Part model, mm, in its own coordinate system. Face numbers are marked on the shaded views. A direction names the side the tool comes from. Coordinates: 2 decimals unless noted, no trailing zeros. Order: outer loops, then holes, each group sorted by start corner. A loop starts at its lowest first (then second) coordinate and runs counter-clockwise, first axis right, second up. Notation, with made-up numbers: (13.25, 61) - (48.25, 61) arc R29 ccw to (48.25, 92) - close; hole circle Ø10 at (-25, 80.25). An arc over 180 degrees is marked (long way). Use a Markdown table: item, result. Add a question column.
1) Saw through at C-C on z = -38.1. List the corners of the cut face in (x, y).
2) Saw through at A-A on y = 13.97. List the corners of the cut face in (x, z) (3 decimals), then the cut area to 3 significant figures.
3) Tool access for the marked faces 4 and 5: list every direction of +Z, -Z, +X, -X, +Y, -Y with a clear straight run to the whole face (end or side of a thin tool).
4) Two-plate mould, pull along Y, no slides. Class the marked faces 1, 2 and 3: +Y half, -Y half, draft (parallel to the pull), parting line (faces both ways), or undercut.
5) Drop a flat-ended pin along its axis: P1, Ø3.5, axis at x = 84.5, y = 15.5, coming from the +Z side. Give the stop position or say it passes through.
6) Saw through at B-B on x = 49. List the corners of the cut face in (y, z) (3 decimals).
7) Wall check: L1, parallel to Y at x = 89, z = -38.1; L2, parallel to Y at x = 69, z = -11 (3 decimals); L3, parallel to Z at x = 87, y = 16.25. Give the ranges that are in metal, low to high. Write a range as [from, to].
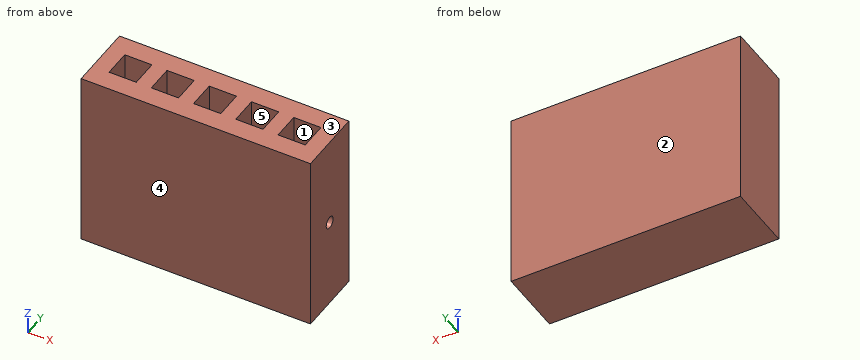
```python
from build123d import *

# Parameters (mm, degrees)
SKETCH1_W           = 96.52
SKETCH1_H           = 76.2
BOSS_EXTRUDE1_DEPTH = 27.94
SKETCH2_W           = 11.43
SKETCH2_H           = 11.43
CUT_EXTRUDE1_DEPTH  = 11.43
SKETCH3_R           = 2.5
CUT_EXTRUDE2_DEPTH  = 12.7


with BuildPart() as part:
    # Sketch1 → Boss-Extrude1 (new body)
    with BuildSketch(Plane(origin=(0, 0, 0), x_dir=(1, 0, 0), z_dir=(0, 1, 0))):
        with Locations((48.26, 38.1)):
            Rectangle(SKETCH1_W, SKETCH1_H)
    extrude(amount=BOSS_EXTRUDE1_DEPTH)

    # Sketch2 → Cut-Extrude1 (cut)
    with BuildSketch(Plane.XY):
        with Locations((12.7, 13.97)):
            Rectangle(SKETCH2_W, SKETCH2_H)
        with Locations((30.48, 13.97)):
            Rectangle(SKETCH2_W, SKETCH2_H)
        with Locations((48.26, 13.97)):
            Rectangle(SKETCH2_W, SKETCH2_H)
        with Locations((66.04, 13.97)):
            Rectangle(SKETCH2_W, SKETCH2_H)
        with Locations((83.82, 13.97)):
            Rectangle(SKETCH2_W, SKETCH2_H)
    extrude(amount=-CUT_EXTRUDE1_DEPTH, mode=Mode.SUBTRACT)

    # Sketch3 → Cut-Extrude2 (cut)
    with BuildSketch(Plane(origin=(96.52, 0, 0), x_dir=(0, 0, -1), z_dir=(1, 0, 0))):
        with Locations((38.1, 13.97)):
            Circle(SKETCH3_R)
    extrude(amount=-CUT_EXTRUDE2_DEPTH, mode=Mode.SUBTRACT)


solid = part.part
```
Results are:
| question | item | result |
|---|---|---|
| 1 | outline | (0, 0) - (96.52, 0) - (96.52, 11.47) - (83.82, 11.47) - (83.82, 16.47) - (96.52, 16.47) - (96.52, 27.94) - (0, 27.94) - close |
| 2 | outline | (0, -76.2) - (96.52, -76.2) - (96.52, -40.6) - (83.82, -40.6) - (83.82, -35.6) - (96.52, -35.6) - (96.52, 0) - (89.535, 0) - (89.535, -11.43) - (78.105, -11.43) - (78.105, 0) - (71.755, 0) - (71.755, -11.43) - (60.325, -11.43) - (60.325, 0) - (53.975, 0) - (53.975, -11.43) - (42.545, -11.43) - (42.545, 0) - (36.195, 0) - (36.195, -11.43) - (24.765, -11.43) - (24.765, 0) - (18.415, 0) - (18.415, -11.43) - (6.985, -11.43) - (6.985, 0) - (0, 0) - close |
| 2 | area | 6,640 mm2 |
| 3 | face 4 | +Z, -Z, +X, -X, -Y |
| 3 | face 5 | +Z |
| 4 | face 1 | undercut |
| 4 | face 2 | +Y half |
| 4 | face 3 | draft |
| 5 | P1 | z = -11.43 |
| 6 | outline | (0, -76.2) - (27.94, -76.2) - (27.94, 0) - (19.685, 0) - (19.685, -11.43) - (8.255, -11.43) - (8.255, 0) - (0, 0) - close |
| 7 | L1 | [0, 11.47], [16.47, 27.94] |
| 7 | L2 | [0, 8.255], [19.685, 27.94] |
| 7 | L3 | [-76.2, -39.13], [-37.07, -11.43] |
